Autodesk Inventor part; units mm, degrees
ref_plane "Work Plane1" through (22, 31.5, 0) normal (0, 0, 1) x (0, 1, 0)
ref_plane "YZ Plane" through (0, 0, 0) normal (1, 0, 0) x (0, 1, 0)
ref_plane "XZ Plane" through (0, 0, 0) normal (0, 1, 0) x (-1, 0, 0)
ref_plane "Work Plane1" through (22, 31.5, 0) normal (0, 0, 1) x (0, 1, 0)
sketch "Sketch1" plane through (22, 31.5, 0) normal (0, 0, 1) x (0, 1, 0)
  line L0 (0, 0) -> (0, 61)
  line L1 (0, 61) -> (-3.5, 61)
  line L2 (-3.5, 0) -> (-3.5, 61)
  circle A0 centre (-5.5, 2) radius 1.75
  circle A1 centre (-28.5, 2) radius 1.75
  line L3 (-3.5, 4) -> (-7.5, 4)
  arc A2 (-8.5, 3) -> (-7.5, 4) centre (-8.5, 4) ccw
  line L4 (-8.5, 3) -> (-21.7679, 3)
  arc A3 (-23.5, 4) -> (-21.7679, 3) centre (-21.7679, 5) ccw
  line L5 (-23.5, 4) -> (-31.5, 4)
  line L6 (-31.5, 0) -> (-31.5, 4)
  line L7 (-3.5, 0) -> (-3.5, 4)
  line L8 (-19.5, 22) -> (-3.5, 22)
  line L9 (-3.5, 22) -> (-3.5, 18)
  line L10 (-19.5, 39) -> (-3.5, 39)
  line L11 (-3.5, 39) -> (-3.5, 43)
  line L12 (-3.5, 57) -> (-6.7679, 57)
  line L13 (-3.5, 61) -> (-3.5, 57)
  line L14 (-3.5, 61) -> (-31.5, 61)
  line L15 (-31.5, 61) -> (-31.5, 57)
  line L16 (-24.004, 57) -> (-31.5, 57)
  line L17 (0, 0) -> (-32.9649, 0)
  line L18 (-32.9649, 0) -> (-32.9649, 61)
  line L19 (-32.9649, 61) -> (0, 61)
  line L20 (0, 61) -> (0, 0)
  line L21 (-3.5, 0) -> (-31.5, 0)
  line L22 (-8.5, 58) -> (-21.7679, 58)
  arc A4 (-7.634, 57.5) -> (-6.7679, 57) centre (-6.7679, 58) ccw
  arc A5 (-24.004, 57) -> (-23.2587, 57.3333) centre (-24.004, 58) ccw
  arc A6 (-21.7679, 58) -> (-23.2587, 57.3333) centre (-21.7679, 56) ccw
  arc A7 (-7.634, 57.5) -> (-8.5, 58) centre (-8.5, 57) ccw
  line L23 (-19.5, 18) -> (-19.5, 22)
  line L24 (-19.5, 18) -> (-3.5, 18)
  line L25 (-19.5, 43) -> (-3.5, 43)
  line L26 (-19.5, 43) -> (-19.5, 39)
  circle A8 centre (-5.5, 59) radius 1.75
  circle A9 centre (-28.5, 59) radius 1.75
  line L27 (-32.9649, 119.5) -> (-32.9649, -58.5)
  point P0 (-3.5, 28.5)
  point P1 (-3.5, 32.5)
  point P2 (-3.5, 61)
  point P3 (-13.5, 58)
  dimension "d25" = 0
  dimension "d26" = 0
extrude "Extrusion1" add sketch "Sketch1" along normal blind 2 contours L17 L2 L1 L0 | L17 L6 L5 A3 L4 A2 L3 L2 | L2 L12 A4 A7 L22 A6 A5 L16 L15 L14 | L3 A2 L4 A3 L5 L6 L17 L18 L19 L15 L16 A5 A6 L22 A7 A4 L12 L2 L25 L26 L10 L8 L23 L24 | L24 L23 L8 L2 | L2 L10 L26 L25 | A0 | A1 | A8 | A9
hole "Hole1" at (20.0645, 2.9032, 2) at (20, 26, 2) at (2, 2.5, 2) at (-19, 2.5, 2) at (-37, 26, 2) at (-37.0645, 2.9032, 2) direction (0, 0, -1) diameter 3.1 end through all countersink diameter 5.8 countersink angle 90
sketch "Sketch4" plane through (22, 31.5, 0) normal (0, 0, -1) x (-1, 0, 0)
  line L0 (39, -19.5) -> (39, -3.5)
  line L1 (39, -3.5) -> (43, -3.5)
  line L2 (43, -19.5) -> (43, -3.5)
  line L3 (43, -19.5) -> (39, -19.5)
  line L4 (22, -19.5) -> (22, -3.5)
  line L5 (18, -19.5) -> (22, -19.5)
  line L6 (18, -19.5) -> (18, -3.5)
  line L7 (22, -3.5) -> (18, -3.5)
  circle A0 centre (20, -29) radius 1.75
  line L8 (22, -31.5) -> (18, -31.5)
  line L9 (18, -31.5) -> (18, -19.5)
  line L10 (22, -19.5) -> (18, -19.5)
  line L11 (22, -19.5) -> (22, -31.5)
  circle A1 centre (41, -29) radius 1.75
  line L12 (39, -31.5) -> (43, -31.5)
  line L13 (39, -19.5) -> (39, -31.5)
  line L14 (39, -23.5) -> (43, -23.5)
  line L15 (43, -31.5) -> (43, -19.5)
  circle A2 centre (59, -5.5) radius 1.75
  circle A3 centre (59, -28.5) radius 1.75
  arc A4 (57, -6.7679) -> (57.5, -7.634) centre (58, -6.7679) ccw
  line L16 (57, -3.5) -> (57, -6.7679)
  line L17 (61, -3.5) -> (57, -3.5)
  line L18 (61, -3.5) -> (61, -31.5)
  line L19 (61, -31.5) -> (57, -31.5)
  line L20 (57, -24.004) -> (57, -31.5)
  arc A5 (57.3333, -23.2587) -> (57, -24.004) centre (58, -24.004) ccw
  arc A6 (57.3333, -23.2587) -> (58, -21.7679) centre (56, -21.7679) ccw
  line L21 (58, -8.5) -> (58, -21.7679)
  arc A7 (58, -8.5) -> (57.5, -7.634) centre (57, -8.5) ccw
  line L22 (61, -32.9649) -> (0, -32.9649)
  line L23 (0, -32.9649) -> (0, 0)
  line L24 (61, -32.9649) -> (0, -32.9649)
  line L25 (0, -32.9649) -> (0, -26.9649)
  line L26 (0, -26.9649) -> (61, -26.9649)
  line L27 (61, -26.9649) -> (61, -32.9649)
  line L28 (61, 0) -> (61, -32.9649)
  line L29 (0, -8.5) -> (61, -8.5)
  line L30 (61, -8.5) -> (61, -2.5)
  line L31 (61, -2.5) -> (0, -2.5)
  line L32 (0, -2.5) -> (0, -8.5)
  circle A8 centre (41, -29) radius 1.55
  line L33 (59, -5.5) -> (41, -29) construction
  line L34 (2, -5.5) -> (20, -29) construction
  circle A9 centre (41, -29) radius 2.9
  circle A10 centre (1.9355, -28.5968) radius 1.55
  line L35 (57, -26.9649) -> (57, -8.5)
  line L36 (4, -26.9649) -> (4, -8.5)
  line L37 (57, -10.5779) -> (44.4482, -26.9649)
  line L38 (54.8127, -8.5) -> (40.6693, -26.9649)
  line L39 (20.3307, -26.9649) -> (6.1873, -8.5)
  line L40 (4, -10.5779) -> (16.5518, -26.9649)
  circle A11 centre (20, -29) radius 2.9
  line L41 (61, -32.9649) -> (0, -32.9649)
  line L42 (0, -32.9649) -> (0, -30.7564)
  line L43 (0, 0) -> (61, 0)
  line L44 (61, 0) -> (61, -3.4)
  circle A12 centre (41, -29) radius 2.9
  arc A13 (61, -26.4372) -> (61, -30.7564) centre (59.0645, -28.5968) ccw
  arc A14 (0, -7.6) -> (0, -3.4) centre (2, -5.5) ccw
  arc A15 (0, -30.7564) -> (0, -26.4372) centre (1.9355, -28.5968) ccw
  arc A16 (61, -3.4) -> (61, -7.6) centre (59, -5.5) ccw
  line L45 (61, -7.6) -> (61, -26.4372)
  line L46 (61, -30.7564) -> (61, -32.9649)
  line L47 (0, -26.4372) -> (0, -7.6)
  line L48 (0, -3.4) -> (0, 0)
  line L49 (61, -3.5) -> (57, -3.5)
  line L50 (61, -3.5) -> (61, -31.5)
  line L51 (61, -31.5) -> (57, -31.5)
  line L52 (57, -3.5) -> (57, -31.5)
  line L53 (4, -26.9649) -> (18, -8.5) construction
  line L54 (57, -26.9649) -> (43, -8.5) construction
  line L55 (57, -24.4822) -> (44.8824, -8.5)
  line L56 (43, -10.9827) -> (55.1176, -26.9649)
  line L57 (5.8824, -26.9649) -> (18, -10.9827)
  line L58 (16.1176, -8.5) -> (4, -24.4822)
  circle A17 centre (41, -29) radius 1.55
  line L59 (22, -8.5) -> (41, -29) construction
  line L60 (39, -8.5) -> (20, -29) construction
  line L61 (39, -24.6355) -> (24.0452, -8.5)
  line L62 (22, -10.7066) -> (37.0687, -26.9649)
  line L63 (23.9313, -26.9649) -> (39, -10.7066)
  line L64 (36.9548, -8.5) -> (22, -24.6355)
  point P0 (42.4697, -31.5)
  point P1 (39.5303, -31.5)
  point P2 (18, -23.9221)
  point P3 (18, -8.5)
  point P4 (22, -8.5)
  point P5 (39, -8.5)
  point P6 (43, -23.9221)
  point P7 (0, -2.5)
  point P8 (28.4548, -17.6711)
  point P9 (30.5, -15.4644)
  point P10 (30.5, -19.8777)
  point P11 (49.8222, -15.0153)
  point P12 (47.9303, -17.4854)
  point P13 (57, -26.5602)
  point P14 (56.6672, -26.9649)
  point P15 (51.7021, -17.4946)
  point P16 (49.8101, -19.9647)
  point P17 (13.0697, -17.4854)
  point P18 (11.1778, -15.0153)
  point P19 (11.1899, -19.9647)
  point P20 (4.3328, -26.9649)
  point P21 (4, -26.5602)
  point P22 (9.2979, -17.4946)
  point P23 (32.5452, -17.6711)
extrude "zeberka" cut sketch "Sketch4" against normal blind 1 contours L13 L61 L63 L0 | L2 L56 L38 L15 | L64 L61 L29 | L62 L26 L63 | L29 L38 L55 | L64 L11 L4 L62 | L56 L26 L37 | L37 L35 L20 L55 | L6 L9 L39 L57 | L58 L39 L29 | L40 L26 L57 | L58 L36 L40
properties part number "back" material "Nylon 6/6"
Source: CAD feature listing. Evaluate the final solid. Frame: model axes, mm. A direction names the side the tool comes from. Round coordinates to 2 decimals unless told otherwise and drop trailing zeros. Loops run counter-clockwise (first coordinate to the right, second up) from the corner with the lowest first, then second, coordinate; pieces in that order, holes last. Notation, with made-up numbers: (34, 65) - (57, 65) arc R26 cw to (57, 97) - close; hole circle Ø11 at (35, -32.5). An arc over 180 degrees is marked (long way). Write item = value, one per line. Start each with the question number.
Item 1: Section query A-A on x = -19. Output: boundary loops of the cut face in (y, z), plus the area to 3 significant figures.
Item 2: Section query C-C on x = -7.5. Output: boundary loops of the cut face in (y, z), plus the area to 3 significant figures.
Item 3: Reachability of faces 1 (the face through (-3.18, 17.36, 0.49)), 2 (the face through (-9, 15, 0)) from +Z, -Z, +X, -X, +Y, -Y: full face, straight path, thin tool, end or side. Return the list, or none.
Item 4: First-contact query: pin 1 Ø3 at (x, y) = (20, 26) entering from +Z; pin 2 Ø1.6 at (x, y) = (15.5, 13) entering from -Z; pin 3 Ø4 at (x, y) = (-37, 26) entering from +Z. Flat tips, straight axial feed; report the tip coordinate or a pass-through.
Item 5: Section query B-B on y = 26. Output: boundary loops of the cut face in (x, z).
Item 6: Material intervals for line 1 (Y direction, x = -37, z = 0.3); line 2 (Y direction, x = 4, z = 1.6); line 3 (Y direction, x = 11, z = 0.15), sorted ascending.
Item 7: Section query D-D on y = 2.5. Count the separate pieces of the cut face and the enclosed holes in it, plus the area to 3 significant figures.
Item 8: Mould query, pull axis Y, two halves, no side actions, for faces 3 (the face through (-33, 14, 1)), 4 (the face through (22, 15, 1)), 5 (the face through (11, 7, 1)). Classes: released by +Y, released by -Y, zero draft, split by the parting line, or undercut.
Results list:
q1.outline = (-1.46, 0) - (0.95, 0) - (0.95, 0.65) - (-0.4, 2) - (-1.46, 2) - close; (4.05, 0) - (31.5, 0) - (31.5, 2) - (5.4, 2) - (4.05, 0.65) - close
q1.area = 57.9 mm²
q2.outline = (-1.46, 0) - (4.54, 0) - (4.54, 1) - (10.54, 1) - (10.54, 0) - (17.11, 0) - (17.11, 1) - (23, 1) - (23, 0) - (31.5, 0) - (31.5, 2) - (-1.46, 2) - close
q2.area = 54.0 mm²
q3.face_1 = -Z
q3.face_2 = -Z, +X, -X, +Y, -Y
q4.pin_1 = through
q4.pin_2 = 1
q4.pin_3 = 1.1
q5.outline = (-39, 0) - (-38.55, 0) - (-38.55, 0.65) - (-39, 1.1) - close; (-35.45, 0) - (18.45, 0) - (18.45, 0.65) - (17.1, 2) - (-34.1, 2) - (-35.45, 0.65) - close; (21.55, 0) - (22, 0) - (22, 1.1) - (21.55, 0.65) - close
q6.line_1 = -1.46 to 1.35, 4.45 to 24.45, 27.55 to 31.5
q6.line_2 = -1.46 to 1, 4 to 31.5
q6.line_3 = -1.46 to 4.54, 11.28 to 16.72, 23 to 31.5
q7.separate_pieces = 5
q7.enclosed_holes = 0
q7.area = 91.1 mm²
q8.face_3 = undercut
q8.face_4 = zero draft
q8.face_5 = undercut
